```python
from build123d import *

# Parameters (mm, degrees)
SKETCH_1_R      = 7.5
EXTRUDE_1_DEPTH = 280
SKETCH_2_R      = 6
EXTRUDE_2_DEPTH = 40
SKETCH_3_R      = 5
EXTRUDE_3_DEPTH = 15
EXTRUDE_START   = 9
SKETCH_4_R      = 5
EXTRUDE_4_DEPTH = 9
SKETCH_5_R      = 4.65
EXTRUDE_5_DEPTH = 1.1
EXTRUDE_START_2 = 3
SKETCH_6_R      = 5
EXTRUDE_6_DEPTH = 3


with BuildPart() as part:
    # 草图1 → 凸台-拉伸1 (new body)
    with BuildSketch(Plane(origin=(0, 0, 0), x_dir=(1, 0, 0), z_dir=(0, 1, 0))):
        with Locations(Location((0, 0, 0), (0, 0, 270))):
            Circle(SKETCH_1_R)
    extrude(amount=EXTRUDE_1_DEPTH)

    # 草图2 → 凸台-拉伸2 (add)
    with BuildSketch(Plane(origin=(0, 280, 0), x_dir=(1, 0, 0), z_dir=(0, 1, 0))):
        with Locations(Location((0, 0, 0), (0, 0, 270))):
            Circle(SKETCH_2_R)
    extrude(amount=EXTRUDE_2_DEPTH)

    # 草图3 → 凸台-拉伸3 (add)
    with BuildSketch(Plane(origin=(0, 320, 0), x_dir=(1, 0, 0), z_dir=(0, 1, 0))):
        with Locations(Location((0, 0, 0), (0, 0, 270))):
            Circle(SKETCH_3_R)
    extrude(amount=EXTRUDE_3_DEPTH)

    # 草图4 → 凸台-拉伸4 (add)
    with BuildSketch(Plane.XZ.offset(EXTRUDE_START)):
        with Locations(Location((0, 0, 0), (0, 0, 90))):
            Circle(SKETCH_4_R)
    extrude(amount=-EXTRUDE_4_DEPTH)

    # 草图5 → 凸台-拉伸5 (add)
    with BuildSketch(Plane.XZ.offset(9)):
        with Locations(Location((0, 0, 0), (0, 0, 270))):
            Circle(SKETCH_5_R)
    extrude(amount=EXTRUDE_5_DEPTH)

    # 草图6 → 凸台-拉伸6 (add)
    with BuildSketch(Plane.XZ.offset(10.1).offset(EXTRUDE_START_2)):
        with Locations(Location((0, 0, 0), (0, 0, 90))):
            Circle(SKETCH_6_R)
    extrude(amount=-EXTRUDE_6_DEPTH)


solid = part.part
```
Model file for the job. Use its own axes, mm. A direction names the side the tool comes from. Round coordinates to 2 decimals unless told otherwise and drop trailing zeros. Order: outer loops, then holes, each group sorted by start corner. A loop starts at its lowest first (then second) coordinate and runs counter-clockwise, first axis right, second up. Notation, with made-up numbers: M -21,85.5 L -12,85.5 A22 cw -12,107.5 Z; hole C 24,60.25 d6. An arc over 180 degrees is marked long. Use CSV: the item, a comma, the result in double quotes.
Item 1: Pull direction Y, two halves, no side cores. Call faces 1 (the face through (0, -13.1, 0)), 2 (the face through (4, 320, -4)), 3 (the face through (1.397, -9.542, -4.435)): released by +Y, released by -Y, zero draft, split by the parting line, or undercut.
Worked answers:
face 1,"released by -Y"
face 2,"released by +Y"
face 3,"undercut"
Item 2: Saw through at D-D (y = 310). List the corners of the cut face in (x, z).
Worked answers:
outline,"C 0,0 d12"
Item 3: Saw through at C-C (y = 167.5). List the corners of the cut face in (x, z).
Worked answers:
outline,"C 0,0 d15"
Item 4: Saw through at B-B (z = 0). List the corners of the cut face in (x, y).
Worked answers:
outline,"M -7.5,0 L -5,0 L -5,-9 L -4.65,-9 L -4.65,-10.1 L -5,-10.1 L -5,-13.1 L 5,-13.1 L 5,-10.1 L 4.65,-10.1 L 4.65,-9 L 5,-9 L 5,0 L 7.5,0 L 7.5,280 L 6,280 L 6,320 L 5,320 L 5,335 L -5,335 L -5,320 L -6,320 L -6,280 L -7.5,280 Z"
Item 5: Saw through at A-A (x = 0). List the corners of the cut face in (y, z).
Worked answers:
outline,"M -13.1,-5 L -10.1,-5 L -10.1,-4.65 L -9,-4.65 L -9,-5 L 0,-5 L 0,-7.5 L 280,-7.5 L 280,-6 L 320,-6 L 320,-5 L 335,-5 L 335,5 L 320,5 L 320,6 L 280,6 L 280,7.5 L 0,7.5 L 0,5 L -9,5 L -9,4.65 L -10.1,4.65 L -10.1,5 L -13.1,5 Z"
Item 6: Pin check, flat tips, straight feed: pin 1 (1 mm diameter, centred on x = 4.5, y = 205, fed in from +Z); pin 2 (8 mm diameter, centred on x = -5.5, y = 124.5, fed in from -Z); pin 3 (3 mm diameter, centred on x = 3, y = 93.5, fed in from +Z). Stop position of each tip, or through.
Worked answers:
pin 1,"z = 6.34"
pin 2,"z = -7.35"
pin 3,"z = 7.35"
Item 7: Which spindle directions (+Z, -Z, +X, -X, +Y, -Y) get a long thin tool onto all of the face, cutting with end or side? Do faces 4 (the face through (4.88, -11.62, -1.08)), 5 (the face through (0, 335, 0)), 6 (the face through (-4.88, 327.4, -1.08)). Say none if no direction does.
Worked answers:
face 4,"-Y"
face 5,"+Z, -Z, +X, -X, +Y"
face 6,"+Y"
Item 8: Probe probe 1 along Y at (x, z) = (-3.25, 3.5); probe 2 along Y at (x, z) = (1.5, -7); probe 3 along Z at (x, y) = (-0.25, 110). List the from-to ranges inside material, lowest first.
Worked answers:
probe 1,"-13.1 to -10.1, -9 to 335"
probe 2,"0 to 280"
probe 3,"-7.5 to 7.5"
